Input: part model. Units: mm. Frame: model coordinates. Face numbers are marked on the shaded views. A direction names the side the tool comes from. Give positions to 0.01 mm unless a question says otherwise; leave off trailing zeros. Loops run counter-clockwise (first coordinate to the right, second up) from the corner with the lowest first, then second, coordinate; pieces in that order, holes last. Notation, with made-up numbers: (85, -36.75) - (128, -36.75) arc R36 ccw to (128, -2.75) - close; hole circle Ø8 at (-26, 25.5). An arc over 180 degrees is marked (long way). Answer as a JSON object with one key per item and string values. Group by question number.
(1) Material intervals for L1, parallel to X at y = -19, z = 0.5; L2, parallel to X at y = -22, z = 0.45; L3, parallel to Y at x = -10, z = 2.9, sorted ascending.
(2) Pin query (flat end, axial travel): P1, Ø1.4, axis at x = -13, z = 2, coming from the -Y side; P2, Ø2, axis at x = 14, z = 3.5, coming from the -Y side; P3, Ø2, axis at y = -19, z = 0.5, coming from the +X side; P4, Ø4, axis at x = 0.5, y = -6.5, coming from the +Z side. Return the tip coordinate at first contact, or that it passes through.
(3) Access query for the marked faces 5 and 6. Directions: +Z, -Z, +X, -X, +Y, -Y. A direction counts if a zero-diameter tool reaches every point of the face in a straight line with its end or side. Return the directions, or none.
(4) Section query A-A (x = -19). Return loops of the section in (y, z), plus the area to 3 significant figures.
(5) Section query C-C (z = 2.9). Count the separate pieces of the cut face and the enclosed holes in it, plus the area to 3 significant figures.
(6) Section query B-B (y = -13.75). Return loops of the section in (x, z).
(7) Section query D-D (x = -4.5). Return loops of the section in (y, z).
(8) Mould query, pull axis X, two halves, no side actions, for the marked faces 1, 2, 3 and 4. Classes: +X half, -X half, draft (parallel to the pull), parting line (faces both ways), or undercut.
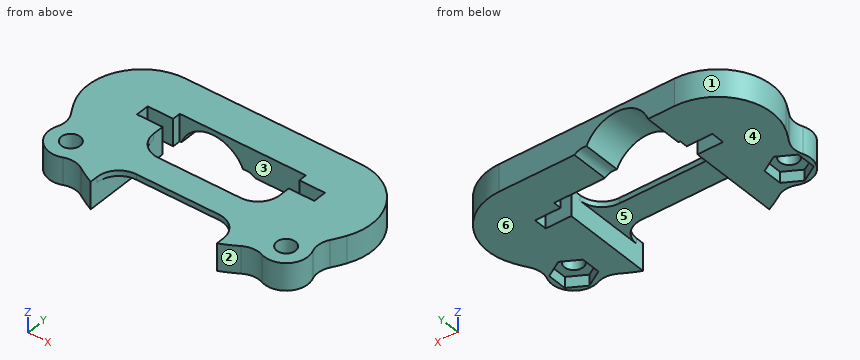
```python
from build123d import *

# Parameters (mm, degrees)
SKETCH1_R           = 1.725
BOSS_EXTRUDE1_DEPTH = 5
CUT_EXTRUDE3_REACH  = 41.552
SKETCH6_W           = 23.2
SKETCH6_H           = 5
BOSS_EXTRUDE2_DEPTH = 1
CUT_EXTRUDE4_DEPTH  = 2
FILLET1_R           = 4
FILLET2_R           = 10


with BuildPart() as part:
    # Sketch1 → Boss-Extrude1 (new body)
    with BuildSketch(Plane.XY):
        with BuildLine():
            Line((-27.928480088, 2), (27.928480088, 2))
            ThreePointArc((27.928480088, 2), (26.866863434, -7.884900077), (22.418161887, -16.775756842))
            ThreePointArc((22.418161887, -16.775756842), (22.627416998, -22.627416998), (16.775756842, -22.418161887))
            ThreePointArc((16.775756842, -22.418161887), (14.270455763, -24.090539478), (11.6, -25.484112698))
            Line((11.6, -25.484112698), (11.6, -8.95))
            Line((11.6, -8.95), (16.3, -8.95))
            Line((16.3, -8.95), (16.3, -6.5))
            Line((16.3, -6.5), (11.6, -6.5))
            Line((11.6, -6.5), (11.6, -5))
            Line((11.6, -5), (-11.6, -5))
            Line((-11.6, -5), (-11.6, -6.5))
            Line((-11.6, -6.5), (-16.3, -6.5))
            Line((-16.3, -6.5), (-16.3, -8.95))
            Line((-16.3, -8.95), (-11.6, -8.95))
            Line((-11.6, -8.95), (-11.6, -25.484112698))
            ThreePointArc((-11.6, -25.484112698), (-14.270455763, -24.090539478), (-16.775756842, -22.418161887))
            ThreePointArc((-16.775756842, -22.418161887), (-22.627416998, -22.627416998), (-22.418161887, -16.775756842))
            ThreePointArc((-22.418161887, -16.775756842), (-26.866863434, -7.884900077), (-27.928480088, 2))
        make_face()
        with Locations((-19.798989873, -19.798989873)):
            Circle(SKETCH1_R, mode=Mode.SUBTRACT)
        with Locations((19.798989873, -19.798989873)):
            Circle(SKETCH1_R, mode=Mode.SUBTRACT)
    extrude(amount=BOSS_EXTRUDE1_DEPTH)

    # Sketch5 → Cut-Extrude3 (cut, up to next)
    with BuildSketch(Plane(origin=(0, 2, 0), x_dir=(1, 0, 0), z_dir=(0, 1, 0)), mode=Mode.PRIVATE) as cut_extrude3_sk1:
        with BuildLine():
            ThreePointArc((0.045901639, 4.540270656), (-11.6, 2), (0.045901639, -0.540270656))
            ThreePointArc((0.045901639, -0.540270656), (3.2, 2), (0.045901639, 4.540270656))
        make_face()
    cut_extrude3_tool1 = extrude(cut_extrude3_sk1.sketch, amount=-CUT_EXTRUDE3_REACH, mode=Mode.PRIVATE) & part.part
    add(cut_extrude3_tool1.solids().sort_by_distance((-4.860102, 2, -2))[0], mode=Mode.SUBTRACT)

    # Sketch6 → Boss-Extrude2 (add)
    with BuildSketch(Plane.XY.offset(5)):
        with Locations((0, -17.5)):
            Rectangle(SKETCH6_W, SKETCH6_H)
    extrude(amount=-BOSS_EXTRUDE2_DEPTH)

    # Sketch7 → Cut-Extrude4 (cut)
    with BuildSketch(Plane(origin=(0, 0, 0), x_dir=(-1, 0, 0), z_dir=(0, 0, -1))):
        Polygon((-16.698989873, -21.588775708), (-16.698989873, -18.009204039), (-19.798989873, -16.219418204), (-22.898989873, -18.009204039), (-22.898989873, -21.588775708), (-19.798989873, -23.378561542), align=None)
        Polygon((22.898989873, -18.009204039), (19.798989873, -16.219418204), (16.698989873, -18.009204039), (16.698989873, -21.588775708), (19.798989873, -23.378561542), (22.898989873, -21.588775708), align=None)
    extrude(amount=-CUT_EXTRUDE4_DEPTH, mode=Mode.SUBTRACT)

    # Fillet1
    fillet1_edges = [part.edges().sort_by_distance(p)[0] for p in [
        (22.418161887, -16.775756842, 2.5),
        (16.775756842, -22.418161887, 2.5),
        (-16.775756842, -22.418161887, 2.5),
        (-22.418161887, -16.775756842, 2.5),
        (-11.6, -20, 4.5),
        (-11.6, -15, 4.5),
        (11.6, -15, 4.5),
        (11.6, -20, 4.5),
    ]]
    fillet(fillet1_edges, radius=FILLET1_R)

    # Fillet2
    fillet2_edges = [part.edges().sort_by_distance(p)[0] for p in [
        (-27.928480088, 2, 2.5),
        (27.928480088, 2, 2.5),
    ]]
    fillet(fillet2_edges, radius=FILLET2_R)


solid = part.part
```
Recorded:
{
 "1": {"L1": "x = -23.72 to -22.9, -16.7 to -11.6, 11.6 to 16.7, 22.9 to 23.72", "L2": "x = -23.14 to -22.19, -17.41 to -11.6, 11.6 to 17.41, 22.19 to 23.14", "L3": "y = -5 to 2"},
 "2": {"P1": "stops at y = -25.15", "P2": "stops at y = -24.8", "P3": "stops at x = 23.8", "P4": "stops at z = 5"},
 "3": {"face 5": "-Z, -Y", "face 6": "-Z, +X, -X, +Y, -Y"},
 "4": {"outline": "(-23.72, 0) - (-22.92, 0) - (-22.92, 2) - (-21.33, 2) - (-21.33, 5) - (-23.72, 5) - close; (-18.27, 2) - (-16.68, 2) - (-16.68, 0) - (1.58, 0) - (1.58, 5) - (-18.27, 5) - close", "area": "105 mm^2"},
 "5": {"separate pieces": "2", "enclosed holes": "2", "area": "716 mm^2"},
 "6": {"outline": "(-24.39, 0) - (-11.6, 0) - (-11.6, 4) - (-10.5, 4) - (-10.5, 5) - (-24.39, 5) - close; (10.5, 4) - (11.6, 4) - (11.6, 0) - (24.39, 0) - (24.39, 5) - (10.5, 5) - close"},
 "7": {"outline": "(-20, 4) - (-15, 4) - (-15, 5) - (-20, 5) - close; (-5, 4.02) - (2, 4.02) - (2, 5) - (-5, 5) - close"},
 "8": {"face 1": "-X half", "face 2": "+X half", "face 3": "undercut", "face 4": "draft"}
}
